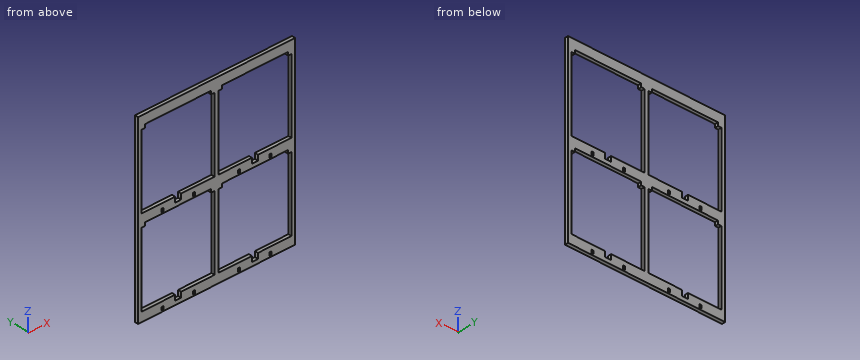
```python
from build123d import *

# Parameters (mm, degrees)
SKETCH1_W                 = 120
SKETCH1_H                 = 145
SKETCH1_W_2               = 109
SKETCH1_H_2               = 117
BOSS_EXTRUDE1_DEPTH       = 5
CUT_EXTRUDE1_DEPTH        = 10
SKETCH5_W                 = 3
SKETCH5_H                 = 5
CUT_EXTRUDE4_DEPTH        = 95.240384125
SKETCH6_W                 = 5
SKETCH6_H                 = 5
BOSS_EXTRUDE2_DEPTH       = 5
LPATTERN1_COUNT           = 2
LPATTERN1_PITCH           = 115
LPATTERN1_COUNT_DIR2      = 2
LPATTERN1_PITCH_DIR2      = 131
LPATTERN1_COPY_1_SKETCH_W = 3
LPATTERN1_COPY_1_SKETCH_H = 5
LPATTERN1_COPY_1_DEPTH    = 95.240384125
LPATTERN1_COPY_2_SKETCH_W = 3
LPATTERN1_COPY_2_SKETCH_H = 5
LPATTERN1_COPY_2_DEPTH    = 95.240384125
LPATTERN1_COPY_3_SKETCH_W = 3
LPATTERN1_COPY_3_SKETCH_H = 5
LPATTERN1_COPY_3_DEPTH    = 95.240384125
LPATTERN1_COPY_4_SKETCH_W = 5
LPATTERN1_COPY_4_SKETCH_H = 5
LPATTERN1_COPY_4_DEPTH    = 5
LPATTERN1_COPY_5_SKETCH_W = 5
LPATTERN1_COPY_5_SKETCH_H = 5
LPATTERN1_COPY_5_DEPTH    = 5
LPATTERN1_COPY_6_SKETCH_W = 5
LPATTERN1_COPY_6_SKETCH_H = 5
LPATTERN1_COPY_6_DEPTH    = 5


with BuildPart() as part:
    # Sketch1 → Boss-Extrude1 (new body)
    with BuildSketch(Plane(origin=(0, 0, 0), x_dir=(1, 0, 0), z_dir=(0, 1, 0))):
        Rectangle(SKETCH1_W, SKETCH1_H)
        Rectangle(SKETCH1_W_2, SKETCH1_H_2, mode=Mode.SUBTRACT)
    boss_extrude1 = extrude(amount=BOSS_EXTRUDE1_DEPTH)

    # Sketch2 → Cut-Extrude1 (cut)
    with BuildSketch(Plane(origin=(0, 5, 0), x_dir=(1, 0, 0), z_dir=(0, 1, 0))):
        Polygon((-4.5, 58.5), (0, 58.5), (4.5, 58.5), (4.5, 66.5), (-4.5, 66.5), align=None)
    cut_extrude1 = extrude(amount=-CUT_EXTRUDE1_DEPTH, mode=Mode.SUBTRACT)

    # Sketch5 → Cut-Extrude4 (cut, through all)
    with BuildSketch(Plane(origin=(0, 5, 0), x_dir=(1, 0, 0), z_dir=(0, 1, 0))):
        with Locations((-23.5, 68)):
            Rectangle(SKETCH5_W, SKETCH5_H)
    cut_extrude4 = extrude(amount=-CUT_EXTRUDE4_DEPTH, mode=Mode.SUBTRACT)

    # Mirror1: Cut-Extrude4 across plane
    add(cut_extrude4.mirror(Plane(origin=(0, 0, 0), x_dir=(0, 0, 1), z_dir=(1, 0, 0))), mode=Mode.SUBTRACT)

    # Sketch6 → Boss-Extrude2 (add)
    with BuildSketch(Plane(origin=(0, 5, 0), x_dir=(1, 0, 0), z_dir=(0, 1, 0))):
        with Locations((52, -56)):
            Rectangle(SKETCH6_W, SKETCH6_H)
    boss_extrude2 = extrude(amount=-BOSS_EXTRUDE2_DEPTH)

    # Mirror2: Boss-Extrude2 across plane
    add(boss_extrude2.mirror(Plane(origin=(0, 0, 0), x_dir=(0, 0, 1), z_dir=(1, 0, 0))))

    # LPattern1: Boss-Extrude1, Cut-Extrude1, Cut-Extrude4, Boss-Extrude2 2 × 2
    with Locations(*[(i * LPATTERN1_PITCH, 0, j * LPATTERN1_PITCH_DIR2) for i in range(LPATTERN1_COUNT) for j in range(LPATTERN1_COUNT_DIR2) if (i, j) != (0, 0)]):
        add(boss_extrude1)
        add(cut_extrude1, mode=Mode.SUBTRACT)
        add(cut_extrude4, mode=Mode.SUBTRACT)
        add(boss_extrude2)

    # LPattern1 copy 1 sketch → LPattern1 copy 1 (cut, through all)
    with BuildSketch(Plane(origin=(0, 5, 131), x_dir=(-1, 0, 0), z_dir=(0, 1, 0))):
        with Locations((-23.5, -68)):
            Rectangle(LPATTERN1_COPY_1_SKETCH_W, LPATTERN1_COPY_1_SKETCH_H)
    extrude(amount=-LPATTERN1_COPY_1_DEPTH, mode=Mode.SUBTRACT)

    # LPattern1 copy 2 sketch → LPattern1 copy 2 (cut, through all)
    with BuildSketch(Plane(origin=(115, 5, 0), x_dir=(-1, 0, 0), z_dir=(0, 1, 0))):
        with Locations((-23.5, -68)):
            Rectangle(LPATTERN1_COPY_2_SKETCH_W, LPATTERN1_COPY_2_SKETCH_H)
    extrude(amount=-LPATTERN1_COPY_2_DEPTH, mode=Mode.SUBTRACT)

    # LPattern1 copy 3 sketch → LPattern1 copy 3 (cut, through all)
    with BuildSketch(Plane(origin=(115, 5, 131), x_dir=(-1, 0, 0), z_dir=(0, 1, 0))):
        with Locations((-23.5, -68)):
            Rectangle(LPATTERN1_COPY_3_SKETCH_W, LPATTERN1_COPY_3_SKETCH_H)
    extrude(amount=-LPATTERN1_COPY_3_DEPTH, mode=Mode.SUBTRACT)

    # LPattern1 copy 4 sketch → LPattern1 copy 4 (add)
    with BuildSketch(Plane(origin=(0, 5, 131), x_dir=(-1, 0, 0), z_dir=(0, 1, 0))):
        with Locations((52, 56)):
            Rectangle(LPATTERN1_COPY_4_SKETCH_W, LPATTERN1_COPY_4_SKETCH_H)
    extrude(amount=-LPATTERN1_COPY_4_DEPTH)

    # LPattern1 copy 5 sketch → LPattern1 copy 5 (add)
    with BuildSketch(Plane(origin=(115, 5, 0), x_dir=(-1, 0, 0), z_dir=(0, 1, 0))):
        with Locations((52, 56)):
            Rectangle(LPATTERN1_COPY_5_SKETCH_W, LPATTERN1_COPY_5_SKETCH_H)
    extrude(amount=-LPATTERN1_COPY_5_DEPTH)

    # LPattern1 copy 6 sketch → LPattern1 copy 6 (add)
    with BuildSketch(Plane(origin=(115, 5, 131), x_dir=(-1, 0, 0), z_dir=(0, 1, 0))):
        with Locations((52, 56)):
            Rectangle(LPATTERN1_COPY_6_SKETCH_W, LPATTERN1_COPY_6_SKETCH_H)
    extrude(amount=-LPATTERN1_COPY_6_DEPTH)


solid = part.part
```
The model under review builds one solid part; all positions refer to its coordinate system, in mm. Coordinates: 2 decimals unless noted, no trailing zeros. Write each loop counter-clockwise with the first axis right and the second up, starting at its lowest first coordinate (ties: lowest second). Pieces come first, ordered by that corner, then holes. Notation, with made-up numbers: (70.5, -2) - (115.5, -2) arc R17 ccw to (115.5, 10) - close; hole circle Ø2 at (87.25, 85). An arc over 180 degrees is marked (long way). Write item = value, one per line.
(1) Consider section A-A, the plane x = -38. Give the boundary of the cut face in (y, z), then the cut area to 3 significant figures.
Result sheet:
outline = (0, -72.5) - (5, -72.5) - (5, -58.5) - (0, -58.5) - close; (0, 58.5) - (5, 58.5) - (5, 72.5) - (0, 72.5) - close; (0, 189.5) - (5, 189.5) - (5, 203.5) - (0, 203.5) - close
area = 210 mm^2
(2) Consider section B-B, the plane z = -25. Give the boundary of the cut face in (x, y).
Result sheet:
outline = (-60, 0) - (-54.5, 0) - (-54.5, 5) - (-60, 5) - close; (54.5, 0) - (60.5, 0) - (60.5, 5) - (54.5, 5) - close; (169.5, 0) - (175, 0) - (175, 5) - (169.5, 5) - close
(3) Consider section C-C, the plane y = 2.85. State how many separate pieces and enclosed holes the cut face has, then the cut area to 3 significant figures.
Result sheet:
separate_pieces = 1
enclosed_holes = 12
area = 13,600 mm^2
(4) For line 1 (Z direction, x = -29, y = 1.65); line 2 (X direction, y = 0.75, z = 188); line 3 (X direction, y = 3.25, z = -46), list the stretches that pass through material, from the lowest coordinate up. Write a range as [from, to].
Result sheet:
line_1 = [-72.5, -58.5], [58.5, 72.5], [189.5, 203.5]
line_2 = [-60, -49.5], [49.5, 65.5], [164.5, 175]
line_3 = [-60, -54.5], [54.5, 60.5], [169.5, 175]
